Here's the drawing with two shaded views (mm, measured from the low corner). I have some questions. A direction names the side the tool comes from. Coordinates: 2 decimals unless noted, no trailing zeros. Order: outer loops, then holes, each group sorted by start corner. A loop starts at its lowest first (then second) coordinate and runs counter-clockwise, first axis right, second up. Notation, with made-up numbers: (29, -31) - (60, -31) arc R21 cw to (60, 7) - close; hole circle Ø10 at (8.5, 19.5). An arc over 180 degrees is marked (long way). Answer as CSV lines item,"result". Start each with the question number.
1. I want a section at B-B, the plane x = 39. List the corners of the cut face in (y, z) for me.
2. I want a section at A-A, the plane y = 12. List the corners of the cut face in (x, z) for me, and give its area (4 significant figures).
3. I need wall thicknesses on probe 1 along Z at (x, y) = (39.5, 9.25); probe 2 along Z at (x, y) = (3, 13); probe 3 along Y at (x, z) = (6.5, 0.5). Which ranges of each line are inside material? Lowest first, please.
4. I want a section at C-C, the plane z = 3.5. List the corners of the cut face in (x, y) for me.
5. I want a section at D-D, the plane y = 8. List the corners of the cut face in (x, z) for me.
6. For the marked faces 1, 2, 3, 4 and 5, which set-ups out of +Z, -Z, +X, -X, +Y, -Y let a thin tool reach every point of the face, with its end or its side?
7. For pin 1 (1.5 mm diameter, centred on x = 18.5, z = 6, fed in from +Y); pin 2 (9 mm diameter, centred on x = 18.5, y = 10.5, fed in from -Z); pin 3 (2.5 mm diameter, centred on x = 3, z = 1, fed in from -Y); pin 4 (6 mm diameter, centred on x = 5.5, y = 12.5, fed in from +Z), each with a flat end and sliding along its axis, tell me the tip position at first contact or that it passes through.
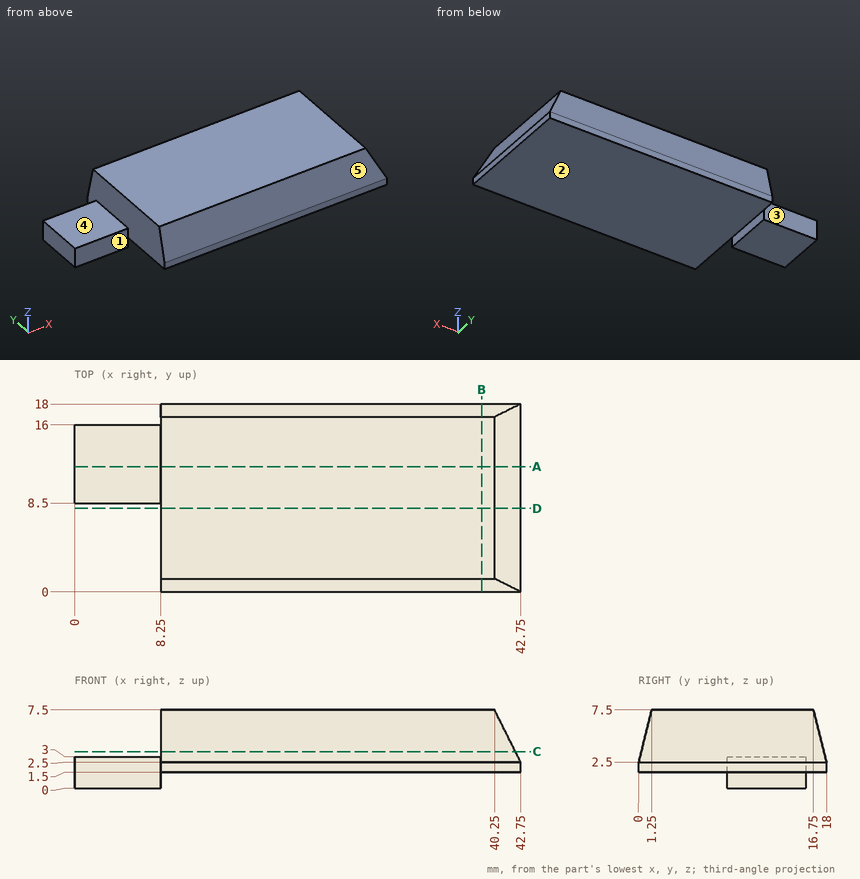
Solved:
1,outline,"(0, 1.5) - (18, 1.5) - (18, 2.5) - (16.75, 7.5) - (1.25, 7.5) - (0, 2.5) - close"
2,outline,"(0, 0) - (8.25, 0) - (8.25, 1.5) - (42.75, 1.5) - (42.75, 2.5) - (40.25, 7.5) - (8.25, 7.5) - (8.25, 3) - (0, 3) - close"
2,area,"225.5 mm2"
3,probe 1,"z = 1.5 to 7.5"
3,probe 2,"z = 0 to 3"
3,probe 3,"y = 8.5 to 16"
4,outline,"(8.25, 0.25) - (42.25, 0.25) - (42.25, 17.75) - (8.25, 17.75) - close"
5,outline,"(8.25, 1.5) - (42.75, 1.5) - (42.75, 2.5) - (40.25, 7.5) - (8.25, 7.5) - close"
6,face 1,"+Z, -Z, -X, -Y"
6,face 2,"-Z, +X, +Y, -Y"
6,face 3,"+Z, -Z, -X, +Y"
6,face 4,"+Z, -X, +Y, -Y"
6,face 5,"+Z, +X, -X, -Y"
7,pin 1,"stops at y = 17.31"
7,pin 2,"stops at z = 1.5"
7,pin 3,"stops at y = 8.5"
7,pin 4,"stops at z = 7.5"
